Could you check a few things on this model? Use its own coordinates, in mm. A direction names the side the tool comes from. Give positions to 0.01 mm unless a question says otherwise; leave off trailing zeros. Order: outer loops, then holes, each group sorted by start corner. A loop starts at its lowest first (then second) coordinate and runs counter-clockwise, first axis right, second up.
from build123d import *

# Parameters (mm, degrees)
BOSS_EXTRUDE1_DEPTH = 2
SKETCH2_R           = 12
BOSS_EXTRUDE2_DEPTH = 2
SKETCH3_R           = 3.85
CUT_EXTRUDE1_DEPTH  = 25
CUT_EXTRUDE2_DEPTH  = 35.465615693
FILLET2_R           = 2
SKETCH6_R           = 1.5
CUT_EXTRUDE3_DEPTH  = 35.29108726


with BuildPart() as part:
    # Sketch1 → Boss-Extrude1 (new body)
    with BuildSketch(Plane(origin=(0, 0, 0), x_dir=(1, 0, 0), z_dir=(0, 1, 0))):
        Polygon((0, 24.378752643), (-17.015462305, 17.117620324), (-24.03237576, 0), (-17.015462305, -17.117620324), (0, -24.378752643), (17.015462305, -17.117620324), (24.03237576, 0), (17.015462305, 17.117620324), align=None)
    extrude(amount=BOSS_EXTRUDE1_DEPTH)

    # Sketch2 → Boss-Extrude2 (add)
    with BuildSketch(Plane(origin=(0, 2, 0), x_dir=(1, 0, 0), z_dir=(0, 1, 0))):
        with Locations(Location((0, 0, 0), (0, 0, 270))):
            Circle(SKETCH2_R)
    extrude(amount=BOSS_EXTRUDE2_DEPTH)

    # Sketch3 → Cut-Extrude1 (cut)
    with BuildSketch(Plane(origin=(0, 4, 0), x_dir=(1, 0, 0), z_dir=(0, 1, 0))):
        with Locations(Location((0, 0, 0), (0, 0, 270))):
            Circle(SKETCH3_R)
    extrude(amount=-CUT_EXTRUDE1_DEPTH, mode=Mode.SUBTRACT)

    # Sketch4 → Cut-Extrude2 (cut, through all)
    with BuildSketch(Plane(origin=(0, 4, 0), x_dir=(1, 0, 0), z_dir=(0, 1, 0))):
        Polygon((0.7, 0), (0.7, 24.080036538), (0, 24.378752643), (-0.7, 24.080036538), (-0.7, 0), align=None)
    extrude(amount=-CUT_EXTRUDE2_DEPTH, mode=Mode.SUBTRACT)

    # Fillet2
    fillet2_edges = [part.edges().sort_by_distance(p)[0] for p in [
        (-11.994890396, 2, 0.350149094),
    ]]
    fillet(fillet2_edges, radius=FILLET2_R - 0.0001)  # a hair under: the kernel refuses the full size

    # Sketch6 → Cut-Extrude3 (cut, through all)
    with BuildSketch(Plane(origin=(0, 2, 0), x_dir=(1, 0, 0), z_dir=(0, 1, 0))):
        with Locations(Location((-18.53237576, 0, 0), (0, 0, 270))):
            Circle(SKETCH6_R)
        with Locations(Location((18.53237576, 0, 0), (0, 0, 270))):
            Circle(SKETCH6_R)
    extrude(amount=-CUT_EXTRUDE3_DEPTH, mode=Mode.SUBTRACT)


solid = part.part
Item 1: For faces 4 (the cylindrical face through (-0.159, 2.028, 3.847)), 5 (the flat face through (0.7, 2, -12)), which set-ups out of +Z, -Z, +X, -X, +Y, -Y let a thin tool reach every point of the face, with its end or its side?
Findings:
face 4: +Y, -Y
face 5: -Z, +Y, -Y
Item 2: Imagine slicing it at A-A on y = 1.45. List the corners of the cut face in (x, z) for me, then the cut area to 3 significant figures.
Findings:
outline: (-24.03, 0) - (-17.02, -17.12) - (-0.7, -24.08) - (-0.7, -3.79) arc R3.85 cw (long way) to (0.7, -3.79) - (0.7, -24.08) - (17.02, -17.12) - (24.03, 0) - (17.02, 17.12) - (0, 24.38) - (-17.02, 17.12) - close; hole circle Ø3 at (-18.53, 0); hole circle Ø3 at (18.53, 0)
area: 1,560 mm2
Item 3: Please list where these lines run through material, in increasing order: line 1 along X through (y, z) = (0.65, 0); line 2 along Y through (x, z) = (-3.5, -17.5); line 3 along X through (y, z) = (1.95, -5.5).
Findings:
line 1: x = -24.03 to -20.03, -17.03 to -3.85, 3.85 to 17.03, 20.03 to 24.03
line 2: y = 0 to 2
line 3: x = -21.78 to -0.7, 0.7 to 21.78
Item 4: For pin 1 (6 mm diameter, centred on x = 18, z = -12.5, fed in from +Y); pin 2 (4.5 mm diameter, centred on x = 0, z = 0, fed in from -Y); pin 3 (1.5 mm diameter, centred on y = 2, z = 18.5, fed in from -X), each with a flat end and sliding along its axis, tell me the tip position at first contact or that it passes through.
Findings:
pin 1: stops at y = 2
pin 2: passes through
pin 3: stops at x = -15.53
Item 5: We'd pull the mould along X, two halves only. Please class faces 1 (the flat face through (10, 2, 11)), 2 (the flat face through (8.39, 0.99, 20.8)), 3 (the flat face through (-0.7, 2, -12)): +X half, -X half, draft (parallel to the pull), parting line (faces both ways), or undercut.
Findings:
face 1: draft
face 2: +X half
face 3: undercut
Item 6: Imagine slicing it at B-B on z = 16.5. List the corners of the cut face in (x, y) for me, then the cut area to 3 significant figures.
Findings:
outline: (-17.27, 0) - (17.27, 0) - (17.27, 2) - (-17.27, 2) - close
area: 69.1 mm2
